Geometry check sheet. Reference: the model listing, model coordinates, mm. Face numbers are marked on the shaded views. A direction names the side the tool comes from. Coordinates: 2 decimals unless noted, no trailing zeros. Write each loop counter-clockwise with the first axis right and the second up, starting at its lowest first coordinate (ties: lowest second). Pieces come first, ordered by that corner, then holes.
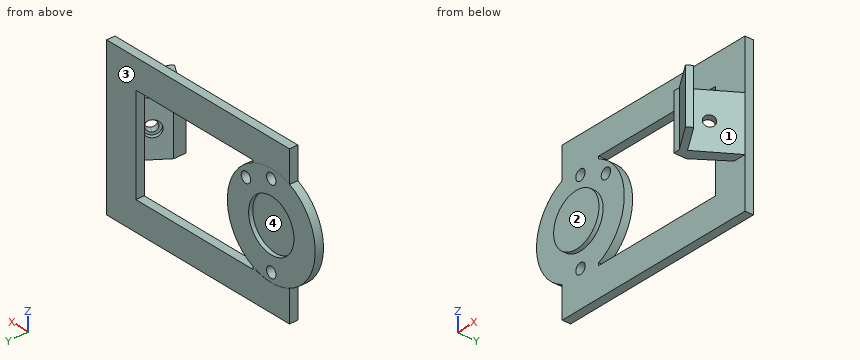
from build123d import *

# Parameters (mm, degrees)
SKETCH1_R           = 30.5
BOSS_EXTRUDE1_DEPTH = 5
SKETCH2_R           = 15.75
CUT_EXTRUDE1_DEPTH  = 2.5
SKETCH3_R           = 15.75
BOSS_EXTRUDE2_DEPTH = 2.5
SKETCH4_R           = 3.25
CUT_EXTRUDE2_DEPTH  = 5.08
SKETCH5_R           = 3.25
CUT_EXTRUDE3_DEPTH  = 5.08
SKETCH6_R           = 3.25
CUT_EXTRUDE4_DEPTH  = 5.08
BOSS_EXTRUDE3_DEPTH = 5.08
BOSS_EXTRUDE4_DEPTH = 5.08
SKETCH9_W           = 17.526
SKETCH9_H           = 5.08
BOSS_EXTRUDE5_DEPTH = 101.6
SKETCH10_W          = 17.526
SKETCH10_H          = 5.08
BOSS_EXTRUDE6_DEPTH = 101.6
SKETCH11_W          = 20.32
SKETCH11_H          = 5.08
BOSS_EXTRUDE7_DEPTH = 63.5
SKETCH12_W          = 20.32
SKETCH12_H          = 33.10825604
BOSS_EXTRUDE8_DEPTH = 25.4
CUT_EXTRUDE5_DEPTH  = 33.274
CUT_EXTRUDE6_DEPTH  = 33.274
SKETCH16_W          = 33.10825604
SKETCH16_H          = 3.81
BOSS_EXTRUDE9_DEPTH = 20.32
CUT_EXTRUDE7_DEPTH  = 7.62
SKETCH20_R          = 4.826
CUT_EXTRUDE9_DEPTH  = 2.54


with BuildPart() as part:
    # Sketch1 → Boss-Extrude1 (new body)
    with BuildSketch(Plane(origin=(0, 0, 0), x_dir=(1, 0, 0), z_dir=(0, 1, 0))):
        with Locations(Location((0, 0, 0), (0, 0, 270))):
            Circle(SKETCH1_R)
    extrude(amount=BOSS_EXTRUDE1_DEPTH)

    # Sketch2 → Cut-Extrude1 (cut)
    with BuildSketch(Plane(origin=(0, 5, 0), x_dir=(1, 0, 0), z_dir=(0, 1, 0))):
        with Locations(Location((0, 0, 0), (0, 0, 270))):
            Circle(SKETCH2_R)
    extrude(amount=-CUT_EXTRUDE1_DEPTH, mode=Mode.SUBTRACT)

    # Sketch3 → Boss-Extrude2 (add)
    with BuildSketch(Plane.XZ):
        with Locations(Location((0, 0, 0), (0, 0, 90))):
            Circle(SKETCH3_R)
    extrude(amount=BOSS_EXTRUDE2_DEPTH)

    # Sketch4 → Cut-Extrude2 (cut)
    with BuildSketch(Plane(origin=(0, 0, 0), x_dir=(-1, 0, 0), z_dir=(0, -1, 0))):
        with Locations(Location((0, 25, 0), (0, 0, 90))):
            Circle(SKETCH4_R)
    extrude(amount=-CUT_EXTRUDE2_DEPTH, mode=Mode.SUBTRACT)

    # Sketch5 → Cut-Extrude3 (cut)
    with BuildSketch(Plane.XZ):
        with Locations(Location((0, 25, 0), (0, 0, 270))):
            Circle(SKETCH5_R)
    extrude(amount=-CUT_EXTRUDE3_DEPTH, mode=Mode.SUBTRACT)

    # Sketch6 → Cut-Extrude4 (cut)
    with BuildSketch(Plane.XZ):
        with Locations(Location((17.674476483, 17.680862, 0), (0, 0, 270))):
            Circle(SKETCH6_R)
    extrude(amount=-CUT_EXTRUDE4_DEPTH, mode=Mode.SUBTRACT)

    # Sketch7 → Boss-Extrude3 (add)
    with BuildSketch(Plane(origin=(0, 0, 0), x_dir=(-1, 0, 0), z_dir=(0, -1, 0))):
        with BuildLine():
            ThreePointArc((12.7, -27.73012802), (6.499272859, -29.79948745), (0, -30.5))
            ThreePointArc((0, -30.5), (-6.499272859, -29.79948745), (-12.7, -27.73012802))
            Line((-12.7, -27.73012802), (-12.7, -46.78012802))
            Line((-12.7, -46.78012802), (12.7, -46.78012802))
            Line((12.7, -46.78012802), (12.7, -27.73012802))
        make_face()
    extrude(amount=-BOSS_EXTRUDE3_DEPTH)

    # Sketch8 → Boss-Extrude4 (add)
    with BuildSketch(Plane.XZ):
        with BuildLine():
            ThreePointArc((0, -30.5), (-6.499272859, -29.79948745), (-12.7, -27.73012802))
            Line((-12.7, -27.73012802), (-12.7, -46.78012802))
            Line((-12.7, -46.78012802), (12.7, -46.78012802))
            Line((12.7, -46.78012802), (12.7, -27.73012802))
            ThreePointArc((12.7, -27.73012802), (6.499272859, -29.79948745), (0, -30.5))
        make_face()
    extrude(amount=-BOSS_EXTRUDE4_DEPTH)

    # Sketch9 → Boss-Extrude5 (add)
    with BuildSketch(Plane(origin=(12.7, 0, 0), x_dir=(0, 0, -1), z_dir=(1, 0, 0))):
        with Locations((38.01712802, 2.54)):
            Rectangle(SKETCH9_W, SKETCH9_H)
    extrude(amount=BOSS_EXTRUDE5_DEPTH)

    # Sketch10 → Boss-Extrude6 (add)
    with BuildSketch(Plane(origin=(12.7, 0, 0), x_dir=(0, 0, -1), z_dir=(1, 0, 0))):
        with Locations((-38.01712802, 2.54)):
            Rectangle(SKETCH10_W, SKETCH10_H)
    extrude(amount=BOSS_EXTRUDE6_DEPTH)

    # Sketch11 → Boss-Extrude7 (add)
    with BuildSketch(Plane(origin=(0, 0, 29.25412802), x_dir=(-1, 0, 0), z_dir=(0, 0, -1))):
        with Locations((-104.14, 2.54)):
            Rectangle(SKETCH11_W, SKETCH11_H)
    extrude(amount=BOSS_EXTRUDE7_DEPTH)

    # Sketch12 → Boss-Extrude8 (add)
    with BuildSketch(Plane.XZ):
        with Locations((104.14, 0)):
            Rectangle(SKETCH12_W, SKETCH12_H)
    extrude(amount=BOSS_EXTRUDE8_DEPTH)

    # Sketch13 → Cut-Extrude5 (cut)
    with BuildSketch(Plane.XY.offset(16.55412802)):
        Polygon((114.3, -25.4), (97.79, -25.4), (114.3, 0), align=None)
    extrude(amount=-CUT_EXTRUDE5_DEPTH, mode=Mode.SUBTRACT)

    # Sketch14 → Cut-Extrude6 (cut)
    with BuildSketch(Plane.XY.offset(16.55412802)):
        Polygon((93.98, 0), (93.98, -17.78), (106.68, 0), align=None)
    extrude(amount=-CUT_EXTRUDE6_DEPTH, mode=Mode.SUBTRACT)

    # Sketch16 → Boss-Extrude9 (add)
    with BuildSketch(Plane(origin=(80.351493849, -52.228471002, 0), x_dir=(0, 0, -1), z_dir=(0.8384436163006371, -0.5449883505954142, 0))):
        with Locations((0, 33.902942951)):
            Rectangle(SKETCH16_W, SKETCH16_H)
    extrude(amount=BOSS_EXTRUDE9_DEPTH)

    # Sketch18 → Cut-Extrude7 (cut)
    with BuildSketch(Plane(origin=(80.351493849, -52.228471002, 0), x_dir=(0, 0, -1), z_dir=(0.8384436163006371, -0.5449883505954142, 0))):
        with BuildLine():
            ThreePointArc((0, 49.269942951), (-3.302, 45.967942951), (0, 42.665942951))
            Line((0, 42.665942951), (0, 49.269942951))
        make_face()
        with BuildLine():
            Line((0, 49.269942951), (0, 42.665942951))
            ThreePointArc((0, 42.665942951), (2.334866591, 43.633076359), (3.302, 45.967942951))
            ThreePointArc((3.302, 45.967942951), (2.334866591, 48.302809542), (0, 49.269942951))
        make_face()
    extrude(amount=-CUT_EXTRUDE7_DEPTH, mode=Mode.SUBTRACT)

    # Sketch20 → Cut-Extrude9 (cut)
    with BuildSketch(Plane(origin=(70.639459459, -50.456756757, 0), x_dir=(0, 0, 1), z_dir=(-0.8137334712067354, 0.5812381937190958, 0))):
        with Locations(Location((0, 49.823352123, 0), (0, 0, 270))):
            Circle(SKETCH20_R)
    extrude(amount=-CUT_EXTRUDE9_DEPTH, mode=Mode.SUBTRACT)


solid = part.part
1. Sectioned sample at A-A, the plane x = 71. Record the boundary of the cut face in (y, z).
Computed values:
outline: (0, -46.78) - (5.08, -46.78) - (5.08, -29.25) - (0, -29.25) - close; (0, 29.25) - (5.08, 29.25) - (5.08, 46.78) - (0, 46.78) - close
2. Gauge pin test, flat ends, axial feed: pin 1 Ø8.5 at (x, z) = (17.67, 17.68) entering from -Y; pin 2 Ø19 at (x, z) = (0, 0) entering from -Y; pin 3 Ø0.8 at (y, z) = (3, -28.5) entering from +X. Record the tip position at first contact, or that the pin passes through.
Computed values:
pin 1: stops at y = 0
pin 2: stops at y = -2.5
pin 3: stops at x = 114.3
3. Access from +Z, -Z, +X, -X, +Y, -Y to the whole of each face (thin tool, end or side, straight path). Record for the marked faces 1 and 2.
Computed values:
face 1: +Z, -Z, +X
face 2: +Z, -Z, -X, -Y
4. Draft check along Z on the marked faces 3 and 4. Enter one of: released by +Z, released by -Z, zero draft, split by the parting line, or undercut.
Computed values:
face 3: zero draft
face 4: undercut
5. Sectioned sample at C-C, the plane z = -39. Record the boundary of the cut face in (x, y).
Computed values:
outline: (-12.7, 0) - (114.3, 0) - (114.3, 5.08) - (-12.7, 5.08) - close
6. Thickness scan on line 1 along X through (y, z) = (3, 0); line 2 along X through (y, z) = (3.7, -25); line 3 along X through (y, z) = (1, -1). Record the ranges inside material, lowest first.
Computed values:
line 1: x = -30.5 to -15.75, 15.75 to 30.5, 93.98 to 114.3
line 2: x = -17.47 to -3.25, 3.25 to 17.47, 93.98 to 114.3
line 3: x = -30.48 to 30.48, 93.98 to 114.3
7. Sectioned sample at B-B, the plane z = 25. Record the boundary of the cut face in (x, y), and give its area (3 significant figures).
Computed values:
outline: (-17.47, 0) - (-3.25, 0) - (-3.25, 5) - (-17.47, 5) - close; (3.25, 0) - (17.47, 0) - (17.47, 5) - (3.25, 5) - close; (93.98, 0) - (114.3, 0) - (114.3, 5.08) - (93.98, 5.08) - close
area: 245 mm2
